Can you work these out from the model? Positions are in its coordinate system, mm. Face numbers are marked on the shaded views. Give positions to 0.01 mm unless a question says otherwise; leave off trailing zeros. Write each loop counter-clockwise with the first axis right and the second up, starting at its lowest first coordinate (ties: lowest second). Pieces come first, ordered by that corner, then holes.
from build123d import *

# Parameters (mm, degrees)
SKETCH_1_W          = 17.278028126
SKETCH_1_H          = 65
SKETCH_1_R          = 3.082023979
SKETCH_1_W_2        = 13.6
SKETCH_1_H_2        = 40.3
EXTRUDE_1_DEPTH     = 1
SKETCH_2_W          = 11.366651046
SKETCH_2_H          = 2.279902362
EXTRUDE_2_DEPTH     = 1.8
EXTRUDE_3_DEPTH     = 65
CUT_EXTRUDE_1_DEPTH = 65
EXTRUDE_4_DEPTH     = 65
CHAMFER_1_SIZE      = 1
CHAMFER_2_SIZE      = 1
CHAMFER_2_SIZE2     = 0.839099631


with BuildPart() as part:
    # 草图1 → 凸台-拉伸1 (new body)
    with BuildSketch(Plane.XY):
        with Locations((-31.11996815, 0)):
            Rectangle(SKETCH_1_W, SKETCH_1_H)
        with Locations((-30.167658157, 23.76)):
            Circle(SKETCH_1_R, mode=Mode.SUBTRACT)
        with Locations((-29.904282539, -3.95)):
            Rectangle(SKETCH_1_W_2, SKETCH_1_H_2, mode=Mode.SUBTRACT)
    extrude(amount=EXTRUDE_1_DEPTH)

    # 草图2 → 凸台-拉伸2 (add)
    with BuildSketch(Plane(origin=(0, 0, 0), x_dir=(-1, 0, 0), z_dir=(0, 0, -1))):
        Polygon((36.267658157, 24.697593501), (36.267658157, 27.721628521), (34.929286678, 29.06), (31.365999463, 29.06), (31.365999463, 28.318477538), (35.267658157, 24.697593501), align=None)
        Polygon((28.825820559, 29.06), (26.391624704, 29.06), (24.367658157, 27.036033454), (24.367658157, 24.969921966), (25.477264987, 24.969921966), (28.825820559, 28.318477538), align=None)
        with Locations((28.887927563, -28.775129659)):
            Rectangle(SKETCH_2_W, SKETCH_2_H)
    extrude(amount=EXTRUDE_2_DEPTH)

    # 草图3 → 凸台-拉伸3 (add)
    with BuildSketch(Plane.XZ.offset(32.5)):
        Polygon((-22.480954087, 1), (-20.997208948, 1), (-21.739081518, 0), (-22.480954087, 0), align=None)
    extrude(amount=-EXTRUDE_3_DEPTH)

    # 草图4 → 切除-拉伸1 (cut)
    with BuildSketch(Plane.XZ.offset(32.5)):
        Polygon((-39.758982213, 0), (-39.058774675, 1), (-39.758982213, 1), align=None)
    extrude(amount=-CUT_EXTRUDE_1_DEPTH, mode=Mode.SUBTRACT)

    # 草图5 → 凸台-拉伸4 (add)
    with BuildSketch(Plane.XZ.offset(32.5)):
        Polygon((-21.739081518, 0), (-21.983150121, -0.34856609), (-22.480954087, 0), align=None)
    extrude(amount=-EXTRUDE_4_DEPTH)

    # 倒角1
    chamfer_1_edges = [part.edges().sort_by_distance(p)[0] for p in [
        (-33.249682136, 23.76, 1),
    ]]
    chamfer(chamfer_1_edges, length=CHAMFER_1_SIZE - 0.0001)  # a hair under: the kernel refuses the full size

    # 倒角2
    chamfer_2_edges = [part.edges().sort_by_distance(p)[0] for p in [
        (-36.704282539, -3.95, 1),
        (-29.904282539, -24.1, 1),
        (-23.104282539, -3.95, 1),
        (-29.904282539, 16.2, 1),
    ]]
    chamfer_2_side = [part.faces().sort_by_distance(p)[0] for p in [
        (-34.924209452, 23.76, 1),
    ]]
    chamfer(chamfer_2_edges, length=CHAMFER_2_SIZE, length2=CHAMFER_2_SIZE2, reference=chamfer_2_side[0])


solid = part.part
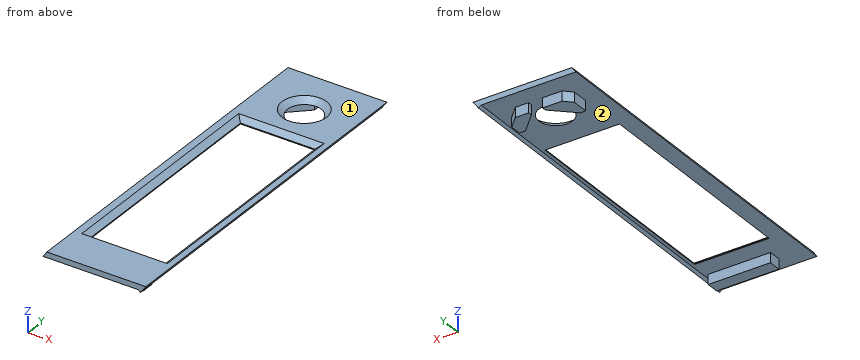
(1) Imagine slicing it at C-C, the plane x = -38.25. Write out the boundary of the cut face in (y, z), plus the area to 3 significant figures.
Returned:
outline: (-32.5, 0) - (32.5, 0) - (32.5, 1) - (-32.5, 1) - close
area: 65.0 mm2
(2) Will these pins go through, and if not, where does the flat tip stop? P1, Ø0.8, axis at x = -36, z = -0.5, coming from the -Y side; P2, Ø4, axis at x = -27.5, y = 13.5, coming from the -Z side; P3, Ø1.4, axis at y = -29, z = -1, coming from the +X side; P4, Ø0.5, axis at y = 26, z = -1, coming from the -X side.
Returned:
P1: stops at y = 24.7
P2: passes through
P3: stops at x = -21.95
P4: stops at x = -36.27
(3) If I drill on L1, parallel to Y at x = -30.25, z = 0.15; L2, parallel to Y at x = -34.5, z = 0.1; L3, parallel to Y at x = -35.5, z = 0.6, over which ranges is the centre line in solid material (lowest first)?
Returned:
L1: y = -32.5 to -24.1, 16.2 to 20.53, 26.99 to 32.5
L2: y = -32.5 to -24.1, 16.2 to 32.5
L3: y = -32.5 to -24.62, 16.72 to 32.5
(4) If we mould it in two halves opening along Y, with no side actions, what happens to the marked faces 1 and 2? For each: +Y half, -Y half, draft (parallel to the pull), parting line (faces both ways), or undercut.
Returned:
face 1: draft
face 2: undercut
(5) Imagine slicing it at B-B, the plane y = 15. Write out the boundary of the cut face in (x, z).
Returned:
outline: (-39.76, 0) - (-36.7, 0) - (-36.7, 0.16) - (-37.7, 1) - (-39.06, 1) - close; (-23.1, 0) - (-22.48, 0) - (-21.98, -0.35) - (-21.74, 0) - (-21, 1) - (-22.1, 1) - (-23.1, 0.16) - close
